Can you work these out from the model? Positions are in its coordinate system, mm. Give positions to 0.01 mm unless a question says otherwise; leave off trailing zeros. Write each loop counter-clockwise with the first axis right and the second up, starting at its lowest first coordinate (ties: lowest second). Pieces come first, ordered by that corner, then holes.
1. Thinking about a two-plate mould opening in X: for faces 1 (the flat face through (36, 60.7, 1)), 2 (the flat face through (72.8, 30, 1)), 3 (the cylindrical face through (71.263, 2.311, 0.739)), which applies, pulls with the +X half, pulls with the -X half, needs draft (parallel to the pull), parting line crosses it, or undercut?
2. Suppose I cut it at C-C (y = 56). Please give me the cut outline in (x, z), and give its area (3 significant figures).
3. Suppose I cut it at A-A (y = 3). Please give me the cut outline in (x, z), and give its area (3 significant figures).
4. Suppose I cut it at B-B (x = 69.6). Please give me the cut outline in (y, z).
5. If I drill on probe 1 along X at (y, z) = (3, 1); probe 2 along Y at (x, z) = (69.6, 1.2); probe 3 along Y at (x, z) = (3, 0.5), over which ranges is the centre line in solid material (lowest first)?
```python
from build123d import *

# Parameters (mm, degrees)
CYLINDER006_R     = 1.8
CYLINDER006_DEPTH = 20
CYLINDER007_R     = 1.8
CYLINDER007_DEPTH = 20
CYLINDER008_R     = 1.8
CYLINDER008_DEPTH = 20
CYLINDER005_R     = 1.8
CYLINDER005_DEPTH = 20
BOX037_W          = 72.8
BOX037_H          = 60.7
BOX037_DEPTH      = 1.5


with BuildPart() as cylinder006:
    # Cylinder006 → Cylinder006 (new body)
    with BuildSketch(Plane(origin=(69.6, 3, 0), x_dir=(1, 0, 0), z_dir=(0, 0, 1))):
        Circle(CYLINDER006_R)
    extrude(amount=CYLINDER006_DEPTH)


with BuildPart() as cylinder007:
    # Cylinder007 → Cylinder007 (new body)
    with BuildSketch(Plane(origin=(3, 56, 0), x_dir=(1, 0, 0), z_dir=(0, 0, 1))):
        Circle(CYLINDER007_R)
    extrude(amount=CYLINDER007_DEPTH)


with BuildPart() as cylinder008:
    # Cylinder008 → Cylinder008 (new body)
    with BuildSketch(Plane(origin=(3, 3, 0), x_dir=(1, 0, 0), z_dir=(0, 0, 1))):
        Circle(CYLINDER008_R)
    extrude(amount=CYLINDER008_DEPTH)


with BuildPart() as fusion010:
    # Cylinder005 → Cylinder005 (new body)
    with BuildSketch(Plane(origin=(69.6, 33, 0), x_dir=(1, 0, 0), z_dir=(0, 0, 1))):
        Circle(CYLINDER005_R)
    extrude(amount=CYLINDER005_DEPTH)

    # Fusion010: union Cylinder006, Cylinder007, Cylinder008
    add(cylinder006.part)
    add(cylinder007.part)
    add(cylinder008.part)


with BuildPart() as fusion010_1:
    # Fusion010 placement: moved
    add(fusion010.part.moved(Location((0, 0, -10))))


with BuildPart() as cut004:
    # Box037 → Box037 (new body)
    with BuildSketch(Plane.XY):
        with Locations((36.4, 30.35)):
            Rectangle(BOX037_W, BOX037_H)
    extrude(amount=BOX037_DEPTH)

    # Cut004: cut Fusion010
    add(fusion010_1.part, mode=Mode.SUBTRACT)


solid = cut004.part
```
Checks:
1. face 1: needs draft
1. face 2: pulls with the +X half
1. face 3: undercut
2. outline: (0, 0) - (1.2, 0) - (1.2, 1.5) - (0, 1.5) - close; (4.8, 0) - (72.8, 0) - (72.8, 1.5) - (4.8, 1.5) - close
2. area: 104 mm2
3. outline: (0, 0) - (1.2, 0) - (1.2, 1.5) - (0, 1.5) - close; (4.8, 0) - (67.8, 0) - (67.8, 1.5) - (4.8, 1.5) - close; (71.4, 0) - (72.8, 0) - (72.8, 1.5) - (71.4, 1.5) - close
3. area: 98.4 mm2
4. outline: (0, 0) - (1.2, 0) - (1.2, 1.5) - (0, 1.5) - close; (4.8, 0) - (31.2, 0) - (31.2, 1.5) - (4.8, 1.5) - close; (34.8, 0) - (60.7, 0) - (60.7, 1.5) - (34.8, 1.5) - close
5. probe 1: x = 0 to 1.2, 4.8 to 67.8, 71.4 to 72.8
5. probe 2: y = 0 to 1.2, 4.8 to 31.2, 34.8 to 60.7
5. probe 3: y = 0 to 1.2, 4.8 to 54.2, 57.8 to 60.7
